from build123d import *

# Parameters (mm, degrees)
BOSS_EXTRUDE1_DEPTH = 3
SKETCH2_R           = 1.25
CUT_EXTRUDE1_DEPTH  = 3


with BuildPart() as part:
    # Sketch1 → Boss-Extrude1 (new body)
    with BuildSketch(Plane.XY):
        Polygon((28.129269299, -5.5398317), (28.129269299, -48.0398317), (25.129269299, -48.0398317), (5.129269299, -48.0398317), (5.129269299, -45.0398317), (-4.870730701, -45.0398317), (-4.870730701, -48.0398317), (-24.870730701, -48.0398317), (-27.870730701, -48.0398317), (-27.870730701, -5.5398317), (-24.870730701, -5.5398317), (-24.870730701, 4.4601683), (-27.870730701, 4.4601683), (-27.870730701, 46.9601683), (-24.870730701, 46.9601683), (-4.870730701, 46.9601683), (-4.870730701, 43.9601683), (5.129269299, 43.9601683), (5.129269299, 46.9601683), (25.129269299, 46.9601683), (28.129269299, 46.9601683), (28.129269299, 4.4601683), (25.129269299, 4.4601683), (25.129269299, -5.5398317), align=None)
    extrude(amount=BOSS_EXTRUDE1_DEPTH)

    # Sketch2 → Cut-Extrude1 (cut)
    with BuildSketch(Plane.XY.offset(3)):
        with Locations((13.629269299, 34.2257933)):
            Circle(SKETCH2_R)
        with Locations((13.629269299, 4.6945433)):
            Circle(SKETCH2_R)
        with Locations((-13.370730701, 34.2257933)):
            Circle(SKETCH2_R)
        with Locations((-13.370730701, 4.6945433)):
            Circle(SKETCH2_R)
    extrude(amount=-CUT_EXTRUDE1_DEPTH, mode=Mode.SUBTRACT)


solid = part.part
CAD build for the part. Positions are in the model's coordinates, mm. A direction names the side the tool comes from. Coordinates: 2 decimals unless noted, no trailing zeros. Order: outer loops, then holes, each group sorted by start corner. A loop starts at its lowest first (then second) coordinate and runs counter-clockwise, first axis right, second up. Notation, with made-up numbers: (-29.5, 6.5) -> (-4.5, 6.5) arc R28 cw to (-4.5, 38.5) -> close; hole circle Ø9 at (25.5, -15). An arc over 180 degrees is marked (long way). Answer in a Markdown table with one row per item.
1) Mould opens along X. For faces 6 (the face through (28.129, 26, 1)), 7 (the face through (27, 4.46, 1)), 8 (the face through (0, -45.04, 1)), 9 (the face through (-4.871, 45, 1)) say: pulls with the +X half, pulls with the -X half, needs draft (parallel to the pull), parting line crosses it, or undercut.
Check values:
| item | result |
|---|---|
| face 6 | pulls with the +X half |
| face 7 | needs draft |
| face 8 | undercut |
| face 9 | undercut |
2) Band-saw the part on A-A (z = 2.55). List the corners of the cut face in (x, y), and give its area (3 significant figures).
Check values:
| item | result |
|---|---|
| outline | (-27.87, -48.04) -> (-4.87, -48.04) -> (-4.87, -45.04) -> (5.13, -45.04) -> (5.13, -48.04) -> (28.13, -48.04) -> (28.13, -5.54) -> (25.13, -5.54) -> (25.13, 4.46) -> (28.13, 4.46) -> (28.13, 46.96) -> (5.13, 46.96) -> (5.13, 43.96) -> (-4.87, 43.96) -> (-4.87, 46.96) -> (-27.87, 46.96) -> (-27.87, 4.46) -> (-24.87, 4.46) -> (-24.87, -5.54) -> (-27.87, -5.54) -> close; hole circle Ø2.5 at (-13.37, 4.69); hole circle Ø2.5 at (-13.37, 34.23); hole circle Ø2.5 at (13.63, 4.69); hole circle Ø2.5 at (13.63, 34.23) |
| area | 5,180 mm2 |
3) Band-saw the part on B-B (y = -3). List the corners of the cut face in (x, z), and give its area (3 significant figures).
Check values:
| item | result |
|---|---|
| outline | (-24.87, 0) -> (25.13, 0) -> (25.13, 3) -> (-24.87, 3) -> close |
| area | 150 mm2 |
4) Drill centre lines: line 1 (Y direction, x = 14.5, z = 0.75); line 2 (Y direction, x = -14.5, z = 1.85); line 3 (Y direction, x = 4, z = 1.4). Where is each one in solid material? Low to high.
Check values:
| item | result |
|---|---|
| line 1 | -48.04 to 3.8, 5.59 to 33.33, 35.12 to 46.96 |
| line 2 | -48.04 to 4.16, 5.23 to 33.69, 34.76 to 46.96 |
| line 3 | -45.04 to 43.96 |
5) Which spindle directions (+Z, -Z, +X, -X, +Y, -Y) get a long thin tool onto all of the face, cutting with end or side? Do faces 1 (the face through (14.784, 4.216, 1.521)), 2 (the face through (1, 0, 3)), 3 (the face through (-26, -5.54, 1)), 4 (the face through (5.129, 45, 1)), 5 (the face through (5.129, -47, 1)). Say none if no direction does.
Check values:
| item | result |
|---|---|
| face 1 | +Z, -Z |
| face 2 | +Z, +X, -X, +Y, -Y |
| face 3 | +Z, -Z, -X |
| face 4 | +Z, -Z, +Y |
| face 5 | +Z, -Z, -Y |
6) Flat gauge pins, fed straight in: P1, Ø2, axis at x = 13.63, y = 34.23, coming from the -Z side; P2, Ø1.5, axis at x = -1.5, z = 2, coming from the -Y side. Where does each tip first touch, or does it go through?
Check values:
| item | result |
|---|---|
| P1 | through |
| P2 | y = -45.04 |
